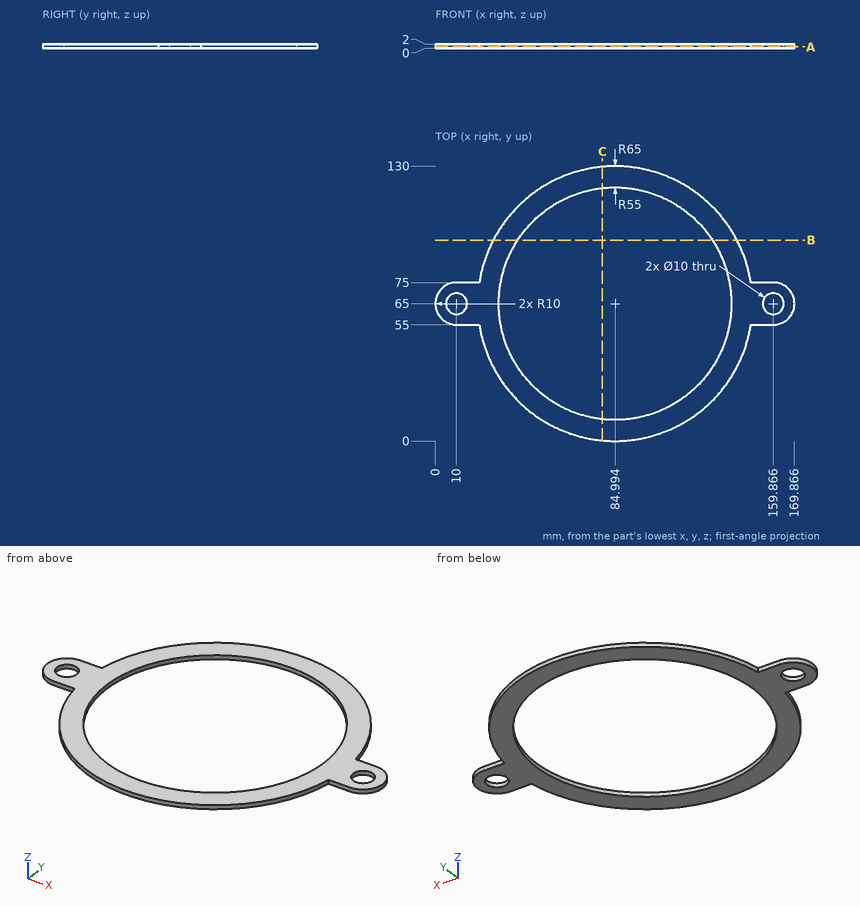
Check sheet for the drawn part. Datum: minimum x, y, z corner. Units: mm. Give positions to 0.01 mm unless a question says otherwise; leave off trailing zeros. Write each loop counter-clockwise with the first axis right and the second up, starting at its lowest first coordinate (ties: lowest second). Pieces come first, ordered by that corner, then holes. Notation, with made-up numbers: M -13.75,24.25 L 3.25,24.25 A25 cw 3.25,50.25 Z; hole C 81.5,-27 d4. An arc over 180 degrees is marked long. One line per question, with ' | ' between items.
1. Cross-section at B-B (y = 95). Enter the section's corners in (x, z).
Ans:
outline: M 27.33,0 L 38.9,0 L 38.9,2 L 27.33,2 Z; M 131.09,0 L 142.66,0 L 142.66,2 L 131.09,2 Z
2. Cross-section at C-C (x = 79). Enter the section's corners in (y, z), plus the area to 3 significant figures.
Ans:
outline: M 0.28,0 L 10.33,0 L 10.33,2 L 0.28,2 Z; M 119.67,0 L 129.72,0 L 129.72,2 L 119.67,2 Z | area: 40.2 mm2
3. Gauge pin test, flat ends, axial feed: pin 1 (8 mm diameter, centred on x = 159.87, y = 65, fed in from -Z); pin 2 (1 mm diameter, centred on y = 58, z = 1.5, fed in from -X); pin 3 (1 mm diameter, centred on x = 42.5, z = 1, fed in from -Y). Record the tip position at first contact, or that the pin passes through.
Ans:
pin 1: through | pin 2: x = 2.4 | pin 3: y = 15.39
4. Cross-section at A-A (z = 0.6). Enter the section's corners in (x, y) (1 decimal).
Ans:
outline: M 10,55 L 20.8,55 A65 ccw 149.2,55 L 159.9,55 A10 ccw 159.9,75 L 149.2,75 A65 ccw 20.8,75 L 10,75 A10 ccw Z; hole C 10,65 d10; hole C 85,65 d110; hole C 159.9,65 d10
5. Scan lines: line 1 along Y through (x, z) = (10, 0.6); line 2 along Y through (x, z) = (103, 0.7) (1 decimal); line 3 along X through (y, z) = (76.5, 1.65). Record each from-to range of solid material in increasing order. Write a range as from..to.
Ans:
line 1: 55..60, 70..75 | line 2: 2.5..13, 117..127.5 | line 3: 21.02..31.21, 138.78..148.97
